from build123d import *

# Parameters (mm, degrees)
BOSS_EXTRUDE1_DEPTH = 40
SKETCH2_W           = 8
SKETCH2_H           = 40
BOSS_EXTRUDE2_DEPTH = 1
CUT_EXTRUDE1_DEPTH  = 5
FILLET1_R           = 0.6
CHAMFER1_SIZE       = 0.4


with BuildPart() as part:
    # Sketch1 → Boss-Extrude1 (new body)
    with BuildSketch(Plane.XY):
        with BuildLine():
            Line((-12.988675135, 0), (0, 0))
            Line((0, 0), (12.988675135, 0))
            ThreePointArc((12.988675135, 0), (14.28771324, 0.75), (14.28771324, 2.25))
            Line((14.28771324, 2.25), (12.7, 5))
            Line((12.7, 5), (6, 5))
            Line((6, 5), (6, 3.565685425))
            ThreePointArc((6, 3.565685425), (6, 3), (5.434314575, 3))
            Line((5.434314575, 3), (-5.434314575, 3))
            ThreePointArc((-5.434314575, 3), (-6, 3), (-6, 3.565685425))
            Line((-6, 3.565685425), (-6, 5))
            Line((-6, 5), (-12.7, 5))
            Line((-12.7, 5), (-14.28771324, 2.25))
            ThreePointArc((-14.28771324, 2.25), (-14.28771324, 0.75), (-12.988675135, 0))
        make_face()
    extrude(amount=-BOSS_EXTRUDE1_DEPTH)

    # Sketch2 → Boss-Extrude2 (add)
    with BuildSketch(Plane.XZ):
        with Locations((0, -20)):
            Rectangle(SKETCH2_W, SKETCH2_H)
    extrude(amount=BOSS_EXTRUDE2_DEPTH)

    # Sketch3 → Cut-Extrude1 (cut, through all)
    with BuildSketch(Plane(origin=(0, 3, 0), x_dir=(1, 0, 0), z_dir=(0, 1, 0))):
        Polygon((0, 3.35), (1.65, 5), (1.65, 35), (0, 36.65), (-1.65, 35), (-1.65, 5), align=None)
    extrude(amount=-CUT_EXTRUDE1_DEPTH, mode=Mode.SUBTRACT)

    # Fillet1
    fillet1_edges = [part.edges().sort_by_distance(p)[0] for p in [
        (-12.7, 5, -20),
        (-6, 5, -20),
        (6, 5, -20),
        (12.7, 5, -20),
    ]]
    fillet(fillet1_edges, radius=FILLET1_R)

    # Chamfer1
    chamfer1_edges = [part.edges().sort_by_distance(p)[0] for p in [
        (-6, 3.982842712, 0),
        (-6, 3, 0),
        (0, 3, 0),
        (6, 3, 0),
        (13.580459161, 3.475, 0),
        (14.28771324, 0.75, 0),
        (14.28771324, 0.75, -40),
        (-8.494337567, 0, 0),
        (-14.28771324, 0.75, 0),
        (13.580459161, 3.475, -40),
        (6, 3, -40),
        (0, 3, -40),
        (8.494337567, 0, 0),
        (8.494337567, 0, -40),
        (4, -0.5, 0),
        (-6, 3, -40),
        (-4, -0.5, -40),
        (4, -0.5, -40),
        (0, -1, 0),
        (0, -1, -40),
        (-6, 3.982842712, -40),
        (-14.28771324, 0.75, -40),
        (9.476794919, 5, 0),
        (9.476794919, 5, -40),
        (6, 3.982842712, 0),
        (-9.476794919, 5, 0),
        (-13.580459161, 3.475, 0),
        (-6.175735931, 4.824264069, 0),
        (-12.653589838, 4.919615242, 0),
        (12.653589838, 4.919615242, 0),
        (6.175735931, 4.824264069, 0),
        (6, 3.982842712, -40),
        (-13.580459161, 3.475, -40),
        (-9.476794919, 5, -40),
        (-6.175735931, 4.824264069, -40),
        (-12.653589838, 4.919615242, -40),
        (12.653589838, 4.919615242, -40),
        (6.175735931, 4.824264069, -40),
        (-8.494337567, 0, -40),
    ]]
    chamfer(chamfer1_edges, length=CHAMFER1_SIZE)


solid = part.part
Verification items for the finished model (mm, model axes). A direction names the side the tool comes from. Coordinates: 2 decimals unless noted, no trailing zeros. Order: outer loops, then holes, each group sorted by start corner. A loop starts at its lowest first (then second) coordinate and runs counter-clockwise, first axis right, second up. Notation, with made-up numbers: M 69.25,25 L 104.25,25 A23 cw 104.25,62 Z; hole C -28,56.25 d3. An arc over 180 degrees is marked long. Return JSON: item names as keys, results as strings.
1) Cross-section at B-B, the plane z = -20.5. Record the boundary of the cut face in (x, y), and give its area (3 significant figures).
Answer list:
{"outline": "M -14.29,2.25 A1.5 ccw -12.99,0 L -4,0 L -4,-1 L -1.65,-1 L -1.65,3 L -5.43,3 A0.4 cw -6,3.57 L -6,4.4 A0.6 ccw -6.6,5 L -12.35,5 A0.6 ccw -12.87,4.7 Z; M 1.65,-1 L 4,-1 L 4,0 L 12.99,0 A1.5 ccw 14.29,2.25 L 12.87,4.7 A0.6 ccw 12.35,5 L 6.6,5 A0.6 ccw 6,4.4 L 6,3.57 A0.4 cw 5.43,3 L 1.65,3 Z", "area": "109 mm2"}
2) Cross-section at A-A, the plane x = 1. Record the boundary of the cut face in (y, z), and give its area (3 significant figures).
Answer list:
{"outline": "M -1,-39.6 L -0.6,-40 L 2.6,-40 L 3,-39.6 L 3,-35.65 L -1,-35.65 Z; M -1,-4.35 L 3,-4.35 L 3,-0.4 L 2.6,0 L -0.6,0 L -1,-0.4 Z", "area": "34.5 mm2"}
3) Thickness scan on L1, parallel to X at y = 1.65, z = -17.5; L2, parallel to X at y = -0.3, z = -17.5; L3, parallel to Y at x = 4.5, z = -5. Record the ranges inside material, lowest first. Write a range as [from, to].
Answer list:
{"L1": "[-14.48, -1.65], [1.65, 14.48]", "L2": "[-4, -1.65], [1.65, 4]", "L3": "[0, 3]"}
4) Cross-section at D-D, the plane z = -4. Record the boundary of the cut face in (x, y), and give its area (3 significant figures).
Answer list:
{"outline": "M -14.29,2.25 A1.5 ccw -12.99,0 L -4,0 L -4,-1 L -0.65,-1 L -0.65,3 L -5.43,3 A0.4 cw -6,3.57 L -6,4.4 A0.6 ccw -6.6,5 L -12.35,5 A0.6 ccw -12.87,4.7 Z; M 0.65,-1 L 4,-1 L 4,0 L 12.99,0 A1.5 ccw 14.29,2.25 L 12.87,4.7 A0.6 ccw 12.35,5 L 6.6,5 A0.6 ccw 6,4.4 L 6,3.57 A0.4 cw 5.43,3 L 0.65,3 Z", "area": "117 mm2"}
5) Gauge pin test, flat ends, axial feed: pin 1 (1 mm diameter, centred on x = -6, z = -14, fed in from +Y); pin 2 (2.5 mm diameter, centred on x = 8.5, z = -25, fed in from -Y); pin 3 (2 mm diameter, centred on y = 0.5, z = -19.5, fed in from +X); pin 4 (0.7 mm diameter, centred on y = 4, z = -24, fed in from -X). Record the tip position at first contact, or that the pin passes through.
Answer list:
{"pin 1": "y = 4.99", "pin 2": "y = 0", "pin 3": "x = 14.49", "pin 4": "x = -13.48"}
6) Cross-section at C-C, the plane x = 11.75. Record the boundary of the cut face in (y, z).
Answer list:
{"outline": "M 0,-39.6 L 0.4,-40 L 4.6,-40 L 5,-39.6 L 5,-0.4 L 4.6,0 L 0.4,0 L 0,-0.4 Z"}
7) Release check for a two-part mould opening along X. For faces 3 (the conical face through (14.03, 0.88, -39.89)), 4 (the flat face through (-13.395, 3.391, -39.803)), 5 (the flat face through (-2, 3, -20)) record: +X half, -X half, draft (parallel to the pull), parting line (faces both ways), or undercut.
Answer list:
{"face 3": "+X half", "face 4": "-X half", "face 5": "undercut"}
8) Access from +Z, -Z, +X, -X, +Y, -Y to the whole of each face (thin tool, end or side, straight path). Record for faces 1 (the flat face through (0.84, 1.03, -35.81)), 2 (the flat face through (0, 2, 0)).
Answer list:
{"face 1": "+Y, -Y", "face 2": "+Z, +X, -X, +Y, -Y"}
